Answer from the drawing. Dimensions are ordinates in mm from the lowest x, y and z of the part. A direction names the side the tool comes from. Coordinates: 2 decimals unless noted, no trailing zeros. Order: outer loops, then holes, each group sorted by start corner. A loop starts at its lowest first (then second) coordinate and runs counter-clockwise, first axis right, second up. Notation, with made-up numbers: (64.5, -24) - (105.5, -24) arc R12 ccw to (105.5, -9) - close; hole circle Ø3 at (21.25, -21). An arc over 180 degrees is marked (long way). Answer as a JSON object with one key per item and string values. Group by question number.
1) Section D-D (y = 95) is taken. Give the vertices of the cut face in (x, z), plus the area to 3 significant figures.
2) Find the intervals of material crossed by line 1 along X through (y, z) = (52, 76); line 2 along X through (y, z) = (73, 57.5); line 3 along Y through (x, z) = (78.5, 54), in increasing order.
3) A tool of negligible diameter and unlimited length cuts with its end or side. For the marked faces 5, 6 and 7, from which of +Z, -Z, +X, -X, +Y, -Y can it reach the whole face along a straight path? Write none if from no direction.
4) Each of these flat-tipped pins is pushed along its axis until it touches: P1, Ø2, axis at y = 62.5, z = 74.5, coming from the -X side; P2, Ø1.5, axis at x = 65.5, y = 41, coming from the -Z side; P3, Ø10.5, axis at x = 52.5, y = 97.5, coming from the +Z side; P4, Ø14, axis at x = 100, y = 68.5, coming from the -Z side. Where does it stop, or does it pass through?
5) Section B-B (y = 69.5) is taken. Give the vertices of the cut face in (x, z) (1 decimal), plus the area to 3 significant figures.
6) The mould has two halves that part along Z. Classify the marked faces 1, 2, 3 and 4: released by +Z, released by -Z, zero draft, split by the parting line, or undercut.
7) Section C-C (x = 7.5) is taken. Give the vertices of the cut face in (y, z).
8) Section A-A (x = 52.5) is taken. Give the vertices of the cut face in (y, z), plus the area to 3 significant figures.
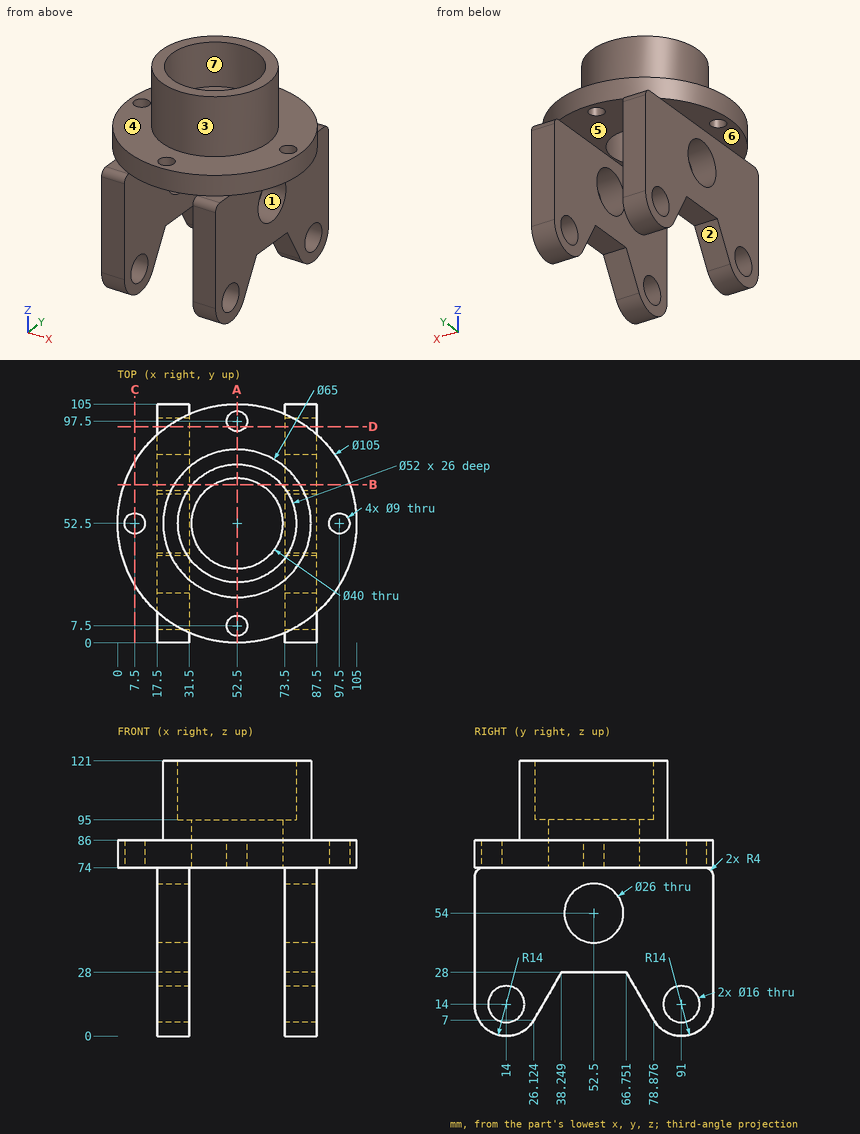
Report:
{
 "1": {"outline": "(17.5, 0.58) - (31.5, 0.58) - (31.5, 7.07) - (17.5, 7.07) - close; (17.5, 20.93) - (31.5, 20.93) - (31.5, 74) - (48.76, 74) - (48.76, 86) - (21.68, 86) - (21.68, 74) - (17.5, 74) - close; (56.24, 74) - (73.5, 74) - (73.5, 20.93) - (87.5, 20.93) - (87.5, 74) - (83.32, 74) - (83.32, 86) - (56.24, 86) - close; (73.5, 0.58) - (87.5, 0.58) - (87.5, 7.07) - (73.5, 7.07) - close", "area": "2,320 mm²"},
 "2": {"line 1": "x = 0 to 3.03, 11.97 to 32.51, 72.49 to 93.03, 101.97 to 105", "line 2": "x = 17.5 to 31.5, 73.5 to 87.5", "line 3": "y = 0 to 39.5, 65.5 to 105"},
 "3": {"face 5": "-Z, +Y, -Y", "face 6": "-Z, -X, +Y, -Y", "face 7": "+Z"},
 "4": {"P1": "stops at x = 0.78", "P2": "passes through", "P3": "stops at z = 86", "P4": "stops at z = 74"},
 "5": {"outline": "(2.8, 74) - (17.5, 74) - (17.5, 23.2) - (31.5, 23.2) - (31.5, 74) - (42, 74) - (42, 95) - (32.8, 95) - (32.8, 121) - (24.8, 121) - (24.8, 86) - (2.8, 86) - close; (63, 74) - (73.5, 74) - (73.5, 23.2) - (87.5, 23.2) - (87.5, 74) - (102.2, 74) - (102.2, 86) - (80.2, 86) - (80.2, 121) - (72.2, 121) - (72.2, 95) - (63, 95) - close", "area": "3,090 mm²"},
 "6": {"face 1": "undercut", "face 2": "released by -Z", "face 3": "zero draft", "face 4": "released by +Z"},
 "7": {"outline": "(25.46, 74) - (48, 74) - (48, 86) - (25.46, 86) - close; (57, 74) - (79.54, 74) - (79.54, 86) - (57, 86) - close"},
 "8": {"outline": "(0, 74) - (3, 74) - (3, 86) - (0, 86) - close; (12, 74) - (32.5, 74) - (32.5, 95) - (26.5, 95) - (26.5, 121) - (20, 121) - (20, 86) - (12, 86) - close; (72.5, 74) - (93, 74) - (93, 86) - (85, 86) - (85, 121) - (78.5, 121) - (78.5, 95) - (72.5, 95) - close; (102, 74) - (105, 74) - (105, 86) - (102, 86) - close", "area": "1,130 mm²"}
}
